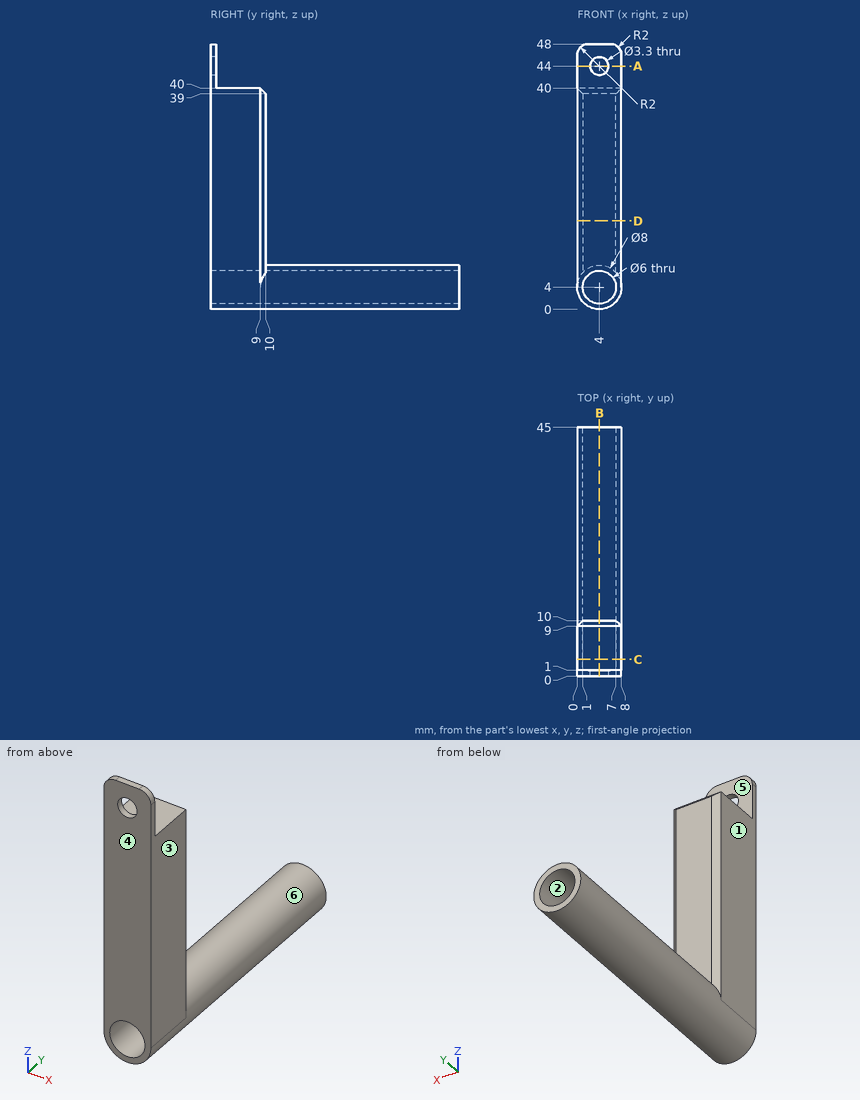
The drawing under review shows one solid part. Ordinate dimensions are in mm from its lowest x, y, z. A direction names the side the tool comes from. Give positions to 0.01 mm unless a question says otherwise; leave off trailing zeros. Order: outer loops, then holes, each group sorted by start corner. A loop starts at its lowest first (then second) coordinate and runs counter-clockwise, first axis right, second up. Notation, with made-up numbers: (0, -37.5) -> (32, -37.5) arc R20 ccw to (32, -3.5) -> close; hole circle Ø9 at (12, -22). An arc over 180 degrees is marked (long way). Write item = value, one per line.
1) We need section B-B, the plane x = 4. Give the boundary of the cut face in (y, z), and give its area (3 significant figures).
Findings:
outline = (0, 0) -> (45, 0) -> (45, 1) -> (0, 1) -> close; (0, 7) -> (45, 7) -> (45, 8) -> (10, 8) -> (10, 39) -> (9, 40) -> (1, 40) -> (1, 42.35) -> (0, 42.35) -> close; (0, 45.65) -> (1, 45.65) -> (1, 48) -> (0, 48) -> close
area = 414 mm^2
2) To check wall thickness, follow L1, parallel to Z at x = 4, y = 35; L2, parallel to Z at x = 4, y = 0.5; L3, parallel to X at y = 0.75, z = 44. State the ranges of each line that lie inside material, in increasing order. Write a range as from..to.
Findings:
L1 = 0..1, 7..8
L2 = 0..1, 7..42.35, 45.65..48
L3 = 0..2.35, 5.65..8
3) For the marked faces 4, 5 and 6, list the 3-axis set-ups (+Z, -Z, +X, -X, +Y, -Y) from which the entire face can be reached by the end or side of a thin tool; tool diameter is ignored.
Findings:
face_4 = +Z, -Z, +X, -X, -Y
face_5 = +Z, +X, -X, +Y
face_6 = +Y
4) We need section A-A, the plane z = 44. Give the boundary of the cut face in (x, y), and give its area (3 significant figures).
Findings:
outline = (0, 0) -> (2.35, 0) -> (2.35, 1) -> (0, 1) -> close; (5.65, 0) -> (8, 0) -> (8, 1) -> (5.65, 1) -> close
area = 4.70 mm^2
5) We need section D-D, the plane z = 16. Give the boundary of the cut face in (x, y), and give its area (3 significant figures).
Findings:
outline = (0, 0) -> (8, 0) -> (8, 9) -> (7, 10) -> (1, 10) -> (0, 9) -> close
area = 79.0 mm^2
6) We need section C-C, the plane y = 3. Give the boundary of the cut face in (x, z).
Findings:
outline = (0, 4) arc R4 ccw to (8, 4) -> (8, 40) -> (0, 40) -> close; hole circle Ø6 at (4, 4)
7) Draft analysis for pull direction X (two halves, no side actions). For the marked faces 1, 2 and 3, state which applies: pulls with the +X half, pulls with the -X half, needs draft (parallel to the pull), parting line crosses it, or undercut.
Findings:
face_1 = pulls with the -X half
face_2 = undercut
face_3 = pulls with the +X half
8) Insertion check: pin 1 (1.8 mm diameter, centred on x = 2.5, z = 20.5, fed in from +Y); pin 2 (4.5 mm diameter, centred on x = 4, z = 44, fed in from +Y); pin 3 (3 mm diameter, centred on x = 2, y = 28, fed in from -Z). Each pin has a flat end and moves straight along its axis. Give the tip position at first contact, or say it passes through.
Findings:
pin_1 = 10
pin_2 = 1
pin_3 = 0.03
